from build123d import *

# Parameters (mm, degrees)
SKETCH1_W                                            = 227.5
SKETCH1_H                                            = 130
BOSS_EXTRUDE1_DEPTH                                  = 5.5
CSK_FOR_M5_HEX_SOCKET_COUNTERSUNK_CAP_SC_D           = 5
CSK_FOR_M5_HEX_SOCKET_COUNTERSUNK_CAP_SC_CSINK_D     = 10.5
CSK_FOR_M5_HEX_SOCKET_COUNTERSUNK_CAP_SC_CSINK_ANGLE = 90
TAP_DRILL_FOR_M5X0_8_TAP1_D                          = 5


with BuildPart() as part:
    # Sketch1 → Boss-Extrude1 (new body)
    with BuildSketch(Plane(origin=(0, 0, 0), x_dir=(0, 0, -1), z_dir=(1, 0, 0))):
        Rectangle(SKETCH1_W, SKETCH1_H)
    extrude(amount=BOSS_EXTRUDE1_DEPTH)

    # CSK for M5 Hex Socket Countersunk Cap Screw1 (through all)
    with Locations(Plane(origin=(5.5, 0, 0), x_dir=(0, 0, -1), z_dir=(1, 0, 0))):
        with Locations((80, 55), (40, 55), (0, 55), (-40, 55), (-80, 55), (-80, -55), (-40, -55), (0, -55), (40, -55), (80, -55)):
            CounterSinkHole(CSK_FOR_M5_HEX_SOCKET_COUNTERSUNK_CAP_SC_D / 2, CSK_FOR_M5_HEX_SOCKET_COUNTERSUNK_CAP_SC_CSINK_D / 2, counter_sink_angle=CSK_FOR_M5_HEX_SOCKET_COUNTERSUNK_CAP_SC_CSINK_ANGLE)

    # Tap Drill for M5x0.8 Tap1 (through all)
    with Locations(Plane(origin=(5.5, 0, 0), x_dir=(0, 0, -1), z_dir=(1, 0, 0))):
        with Locations((-63.75, -52.653836842), (-18.75, -52.653836842), (18.75, -52.653836842), (63.75, -52.653836842)):
            Hole(TAP_DRILL_FOR_M5X0_8_TAP1_D / 2)


solid = part.part
Could you check a few things on this model? Use its own coordinates, in mm. Coordinates: 2 decimals unless noted, no trailing zeros. Order: outer loops, then holes, each group sorted by start corner. A loop starts at its lowest first (then second) coordinate and runs counter-clockwise, first axis right, second up.
Q1. Suppose I cut it at A-A on z = -40. Please give me the cut outline in (x, y).
Q2. Please list where these lines run through material, in increasing order: L1, parallel to Z at x = 2.2, y = 55; L2, parallel to Y at x = 1.3, z = 0; L3, parallel to Z at x = 4.45, y = 54.
Q3. Thinking about a two-plate mould opening in Y: for faces 1 (the flat face through (3, 65, 2)), 2 (the cylindrical face through (1.36, -57.44, -0.54)), 3 (the flat face through (0, 1, 2)), which applies, released by +Y, released by -Y, zero draft, split by the parting line, or undercut?
Q4. Suppose I cut it at C-C on z = 63.75. Please give me the cut outline in (x, y).
Q5. Suppose I cut it at B-B on y = 55. Give the number of separate pieces and of enclosed holes in the cut face, and give its area (3 significant figures).
Q6. Will these pins go through, and if not, where does the flat tip stop? pin 1 (4.5 mm diameter, centred on y = 55, z = 0, fed in from +X); pin 2 (6 mm diameter, centred on y = 55, z = 80, fed in from -X); pin 3 (6.5 mm diameter, centred on y = -55, z = -40, fed in from +X); pin 4 (8 mm diameter, centred on y = 55, z = 40, fed in from +X).
Answer:
1. outline: (0, -65) - (5.5, -65) - (5.5, -60.25) - (2.75, -57.5) - (0, -57.5) - close; (0, -52.5) - (2.75, -52.5) - (5.5, -49.75) - (5.5, 49.75) - (2.75, 52.5) - (0, 52.5) - close; (0, 57.5) - (2.75, 57.5) - (5.5, 60.25) - (5.5, 65) - (0, 65) - close
2. L1: z = -113.75 to -82.5, -77.5 to -42.5, -37.5 to -2.5, 2.5 to 37.5, 42.5 to 77.5, 82.5 to 113.75
2. L2: y = -65 to -57.5, -52.5 to 52.5, 57.5 to 65
2. L3: z = -113.75 to -84.08, -75.92 to -44.08, -35.92 to -4.08, 4.08 to 35.92, 44.08 to 75.92, 84.08 to 113.75
3. face 1: released by +Y
3. face 2: undercut
3. face 3: zero draft
4. outline: (0, -65) - (5.5, -65) - (5.5, -55.15) - (0, -55.15) - close; (0, -50.15) - (5.5, -50.15) - (5.5, 65) - (0, 65) - close
5. separate pieces: 6
5. enclosed holes: 0
5. area: 1,080 mm2
6. pin 1: passes through
6. pin 2: stops at x = 0
6. pin 3: stops at x = 3.5
6. pin 4: stops at x = 4.25
